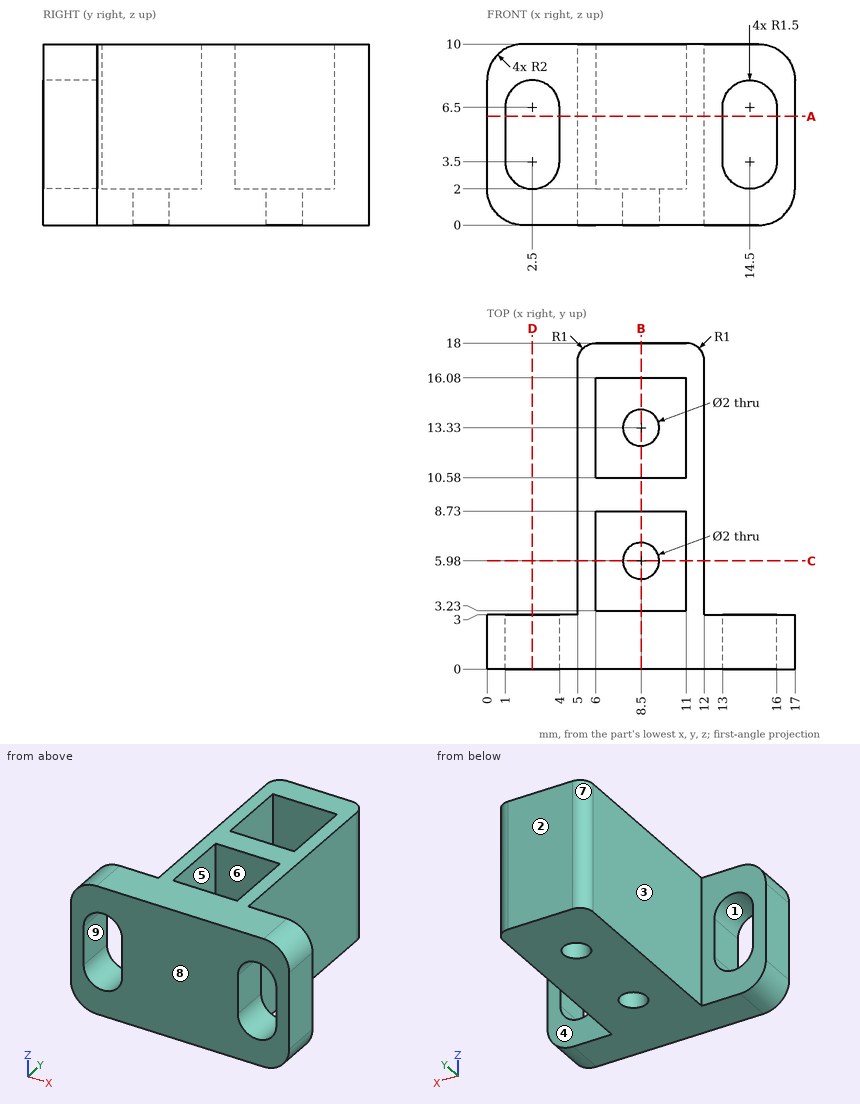
Geometry check sheet. Reference: drawing and pictorial views, mm from the part's lowest x, y, z. A direction names the side the tool comes from. Coordinates: 2 decimals unless noted, no trailing zeros. Loops run counter-clockwise (first coordinate to the right, second up) from the corner with the lowest first, then second, coordinate; pieces in that order, holes last.
1) Material ranges on probe 1 along X at (y, z) = (1.5, 5.25); probe 2 along Y at (x, z) = (6.25, 5); probe 3 along Y at (x, z) = (8.5, 0.75), recorded low to high.
2) Sectioned sample at D-D (x = 2.5). Record the boundary of the cut face in (y, z), and give its area (3 significant figures).
3) Sectioned sample at A-A (z = 6). Record the boundary of the cut face in (x, y), and give its area (3 significant figures).
4) Gauge pin test, flat ends, axial feed: pin 1 (2.5 mm diameter, centred on x = 8.5, y = 5.98, fed in from +Z); pin 2 (1 mm diameter, centred on x = 5, z = 7, fed in from +Y); pin 3 (2.5 mm diameter, centred on x = 14.5, z = 7.5, fed in from +Y). Record the tip position at first contact, or that the pin passes through.
5) Access from +Z, -Z, +X, -X, +Y, -Y to the whole of each face (thin tool, end or side, straight path). Record for the marked faces 1, 2, 3, 4 and 5.
6) Sectioned sample at C-C (y = 5.98). Record the boundary of the cut face in (x, z).
7) Sectioned sample at B-B (x = 8.5). Record the boundary of the cut face in (y, z).
8) Release check for a two-part mould opening along Y. For the marked faces 6, 7, 8 and 9 record: released by +Y, released by -Y, zero draft, split by the parting line, or undercut.
Check sheet entries:
1. probe 1: x = 0 to 1, 4 to 13, 16 to 17
1. probe 2: y = 0 to 3.23, 8.73 to 10.58, 16.08 to 18
1. probe 3: y = 0 to 4.98, 6.98 to 12.33, 14.33 to 18
2. outline: (0, 0) - (3, 0) - (3, 2) - (0, 2) - close; (0, 8) - (3, 8) - (3, 10) - (0, 10) - close
2. area: 12.0 mm2
3. outline: (0, 0) - (1, 0) - (1, 3) - (0, 3) - close; (4, 0) - (13, 0) - (13, 3) - (12, 3) - (12, 17) arc R1 ccw to (11, 18) - (6, 18) arc R1 ccw to (5, 17) - (5, 3) - (4, 3) - close; (16, 0) - (17, 0) - (17, 3) - (16, 3) - close; hole (6, 3.23) - (11, 3.23) - (11, 8.73) - (6, 8.73) - close; hole (6, 10.58) - (11, 10.58) - (11, 16.08) - (6, 16.08) - close
3. area: 82.6 mm2
4. pin 1: stops at z = 2
4. pin 2: stops at y = 17.87
4. pin 3: stops at y = 3
5. face 1: +Y, -Y
5. face 2: +Z, -Z, +X, -X, +Y
5. face 3: +Z, -Z, -X, +Y
5. face 4: +Z, -Z, +X, +Y
5. face 5: +Z
6. outline: (5, 0) - (7.5, 0) - (7.5, 2) - (6, 2) - (6, 10) - (5, 10) - close; (9.5, 0) - (12, 0) - (12, 10) - (11, 10) - (11, 2) - (9.5, 2) - close
7. outline: (0, 0) - (4.98, 0) - (4.98, 2) - (3.23, 2) - (3.23, 10) - (0, 10) - close; (6.98, 0) - (12.33, 0) - (12.33, 2) - (10.58, 2) - (10.58, 10) - (8.73, 10) - (8.73, 2) - (6.98, 2) - close; (14.33, 0) - (18, 0) - (18, 10) - (16.08, 10) - (16.08, 2) - (14.33, 2) - close
8. face 6: undercut
8. face 7: released by +Y
8. face 8: released by -Y
8. face 9: zero draft
